Here's the drawing with two shaded views (mm, measured from the low corner). I have some questions. A direction names the side the tool comes from. Coordinates: 2 decimals unless noted, no trailing zeros. Write each loop counter-clockwise with the first axis right and the second up, starting at its lowest first coordinate (ties: lowest second). Pieces come first, ordered by that corner, then holes. Notation, with made-up numbers: M 75.5,14 L 79.5,14 A25 ccw 79.5,43 Z; hole C 62.25,43.5 d1. An arc over 180 degrees is marked long. Use one line per item in the form item = value. Start each with the question number.
1. Thinking about a two-plate mould opening in Y: for the marked faces 6, 7, 8 and 9, which applies, released by +Y, released by -Y, zero draft, split by the parting line, or undercut?
2. I want a section at B-B, the plane y = 7.5. List the corners of the cut face in (x, z) for me.
3. I want a section at D-D, the plane x = 6.75. List the corners of the cut face in (y, z) for me.
4. On a 3-axis mill with a long thin cutter (end or side, diameter ignored), from which of +Z, -Z, +X, -X, +Y, -Y can I reach the whole of each face in a straight line? I mean the marked faces 1, 2, 3, 4 and 5. Say none if no direction works.
5. I want a section at A-A, the plane z = 0.8. Count the separate pieces of the cut face and the enclosed holes in it.
6. I'm going to push flat-ended pins straight in: pin 1 Ø0.8 at (x, z) = (10, 1) entering from +Y; pin 2 Ø0.8 at (y, z) = (10.5, 0.5) entering from +X. Where does each tip first touch, or does it pass through?
7. Please list where these lines run through material, in increasing order: line 1 along X through (y, z) = (5, 0.55) (1 decimal); line 2 along Z through (x, y) = (4.5, 7.25); line 3 along X through (y, z) = (8.5, 0.5). Write a range as [from, to].
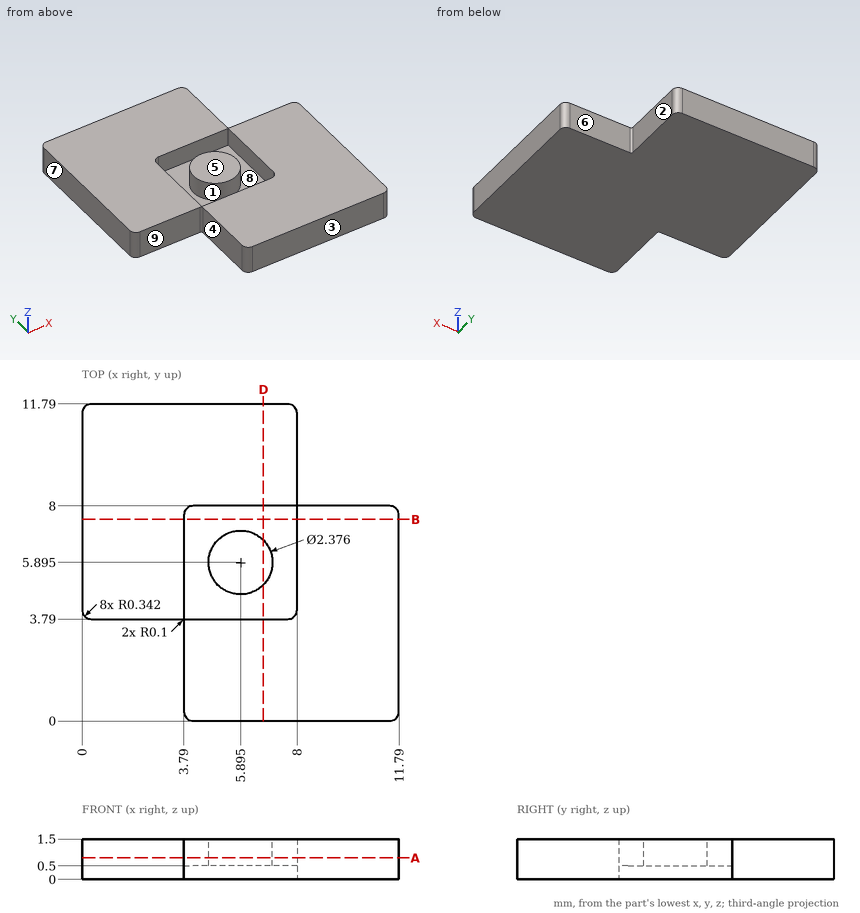
Answer list:
q1.face_6 = released by +Y
q1.face_7 = zero draft
q1.face_8 = undercut
q1.face_9 = released by -Y
q2.outline = M 0,0 L 11.79,0 L 11.79,1.5 L 8,1.5 L 8,0.5 L 3.79,0.5 L 3.79,1.5 L 0,1.5 Z
q3.outline = M 0,0 L 11.79,0 L 11.79,1.5 L 8,1.5 L 8,0.5 L 6.72,0.5 L 6.72,1.5 L 5.07,1.5 L 5.07,0.5 L 3.79,0.5 L 3.79,1.5 L 0,1.5 Z
q4.face_1 = +Z
q4.face_2 = +Z, -Z, +X, +Y
q4.face_3 = +Z, -Z, +X, -X, -Y
q4.face_4 = +Z, -Z, -X, -Y
q4.face_5 = +Z, +X, -X, +Y, -Y
q5.separate_pieces = 2
q5.enclosed_holes = 1
q6.pin_1 = 8
q6.pin_2 = 8
q7.line_1 = [0, 3.8], [5.1, 6.7], [8, 11.8]
q7.line_2 = [0, 0.5]
q7.line_3 = [0, 8]
